```python
from build123d import *

# Parameters (mm, degrees)
F0_W        = 15.9461647272
F0_H        = 30.12368083
F1_DEPTH    = 82.5116038322
F2_T1_DEPTH = 236.0281493159
F3_T        = -2.54


# Not quite as in the source:
# - a fillet or chamfer that OpenCascade refuses, or shapes differently, is made with other operations: its cross-section is extruded or revolved along the edge and cut away or added


with BuildPart() as f1:
    # F0 (on Top) → F1 (new body)
    with BuildSketch(Plane.XY):
        with Locations((7.9730823636, 33.8614284992)):
            Rectangle(F0_W, F0_H)
    extrude(amount=F1_DEPTH)

    # F2: fillet of radius 61.1478122974 on 2 edges, made by hand

    # F2_s2 → F2_t1 (cut)
    with BuildSketch(Plane.XZ.offset(-151.8755031572)):
        with BuildLine():
            ThreePointArc((15.9461647272, 41.3307101351), (11.8204394221, 63.4109398395), (0, 82.5116038322))
            Line((0, 82.5116038322), (0.9040329514, 83.3352217062))
            ThreePointArc((0.9040329514, 83.3352217062), (7.9730823636, 83.7345600782), (15.9461647272, 83.7345600782))
            Line((15.9461647272, 83.7345600782), (17.1691209732, 82.5116038322))
            Line((17.1691209732, 82.5116038322), (17.1691209732, 41.3307101351))
            Line((17.1691209732, 41.3307101351), (15.9461647272, 41.3307101351))
        make_face()
        with BuildLine():
            ThreePointArc((15.9461647272, 41.1808936972), (11.8204394221, 19.1006639927), (0, 0))
            Line((0, 0), (0.9040329514, -0.8236178739))
            ThreePointArc((0.9040329514, -0.8236178739), (7.9730823636, -1.2229562459), (15.9461647272, -1.2229562459))
            Line((15.9461647272, -1.2229562459), (17.1691209732, 0))
            Line((17.1691209732, 0), (17.1691209732, 41.1808936972))
            Line((17.1691209732, 41.1808936972), (15.9461647272, 41.1808936972))
        make_face()
    extrude(amount=F2_T1_DEPTH, mode=Mode.SUBTRACT)

    # F3
    f3_openings = [f1.faces().sort_by_distance(p)[0] for p in [
        (6.459613, 18.799588, 41.255802),
    ]]
    offset(amount=F3_T, openings=f3_openings)


solid = f1.part
```
The model under review builds one solid part; all positions refer to its coordinate system, in mm. A direction names the side the tool comes from. Round coordinates to 2 decimals unless told otherwise and drop trailing zeros. Order: outer loops, then holes, each group sorted by start corner. A loop starts at its lowest first (then second) coordinate and runs counter-clockwise, first axis right, second up. Notation, with made-up numbers: M -7.5,53 L 15.5,53 A10 cw 15.5,71 Z; hole C 89,66 d11. An arc over 180 degrees is marked long. Use a Markdown table: item, result.
1) Draft analysis for pull direction Z (two halves, no side actions). For faces 3 (the face through (10.7, 32.78, 58.93)), 4 (the face through (6, 48.923, 41)), 5 (the face through (11.934, 34.072, 19.396)), state which applies: released by +Z, released by -Z, zero draft, split by the parting line, or undercut.
Report:
| item | result |
|---|---|
| face 3 | undercut |
| face 4 | zero draft |
| face 5 | released by -Z |
2) Consider section D-D (x = 14.5). Write out the cut boundary in (y, z).
Report:
| item | result |
|---|---|
| outline | M 18.8,27.96 L 48.92,27.96 L 48.92,54.55 L 18.8,54.55 Z |
3) Wall thickness on line 1 along X through (y, z) = (33, 41); line 2 along X through (y, z) = (34, 15); line 3 along Z through (x, y) = (6.5, 44): over which ranges is each line inside the solid? List them lowest first. Write a range as [from, to].
Report:
| item | result |
|---|---|
| line 1 | [0, 2.54], [13.41, 15.95] |
| line 2 | [0, 2.54], [7.23, 10.06] |
| line 3 | [8.53, 13.58], [68.93, 73.98] |
4) Consider section C-C (x = 8.75). Write out the cut boundary in (y, z), then the cut area to 3 significant figures.
Report:
| item | result |
|---|---|
| outline | M 18.8,12.4 L 48.92,12.4 L 48.92,70.11 L 18.8,70.11 L 18.8,64.22 L 46.38,64.22 L 46.38,18.29 L 18.8,18.29 Z |
| area | 471 mm^2 |
5) Consider section B-B (z = 15). Write out the cut boundary in (x, y).
Report:
| item | result |
|---|---|
| outline | M 0,18.8 L 2.54,18.8 L 2.54,46.38 L 7.23,46.38 L 7.23,18.8 L 10.06,18.8 L 10.06,48.92 L 0,48.92 Z |
6) Insertion check: pin 1 (8 mm diameter, centred on y = 38, z = 64, fed in from +X); pin 2 (3 mm diameter, centred on x = 12, y = 37, fed in from -Z). Each pin has a flat end and moves straight along its axis. Give the tip position at first contact, or say it passes through.
Report:
| item | result |
|---|---|
| pin 1 | x = 13.03 |
| pin 2 | z = 15.95 |
7) Consider section A-A (y = 28.5). Write out the cut boundary in (x, z).
Report:
| item | result |
|---|---|
| outline | M 0,0 A61.15 ccw 15.95,41.18 L 15.95,41.33 A61.15 ccw 0,82.51 Z; hole M 2.54,7.19 A58.61 ccw 13.41,41.18 L 13.41,41.33 A58.61 ccw 2.54,75.32 Z |
8) Tool access review of faces 1 (the face through (0, 34, 41)), 2 (the face through (7, 46.383, 41)): name each direction out of +Z, -Z, +X, -X, +Y, -Y from which nothing blocks a thin tool from reaching the whole face with its end or side.
Report:
| item | result |
|---|---|
| face 1 | +Z, -Z, -X, +Y, -Y |
| face 2 | -Y |
